Can you work these out from the model? Positions are in its coordinate system, mm. A direction names the side the tool comes from. Give positions to 0.01 mm unless a question says otherwise; leave off trailing zeros. Write each loop counter-clockwise with the first axis right and the second up, starting at its lowest first coordinate (ties: lowest second). Pieces come first, ordered by that corner, then holes. Notation, with made-up numbers: M 2,44 L 24,44 A14 cw 24,70 Z; hole C 51.5,73 d6. An arc over 180 degrees is marked long. Write each question's results on one line, items separated by ' | '.
from build123d import *

# Parameters (mm, degrees)
F1_R     = 2.5
F3_DEPTH = 35
F4_R     = 0.882114
F4_R_2   = 0.903169
F5_DEPTH = 25


with BuildPart() as f2:
    # F2: sweep along a path in F0
    with BuildLine(Plane.YZ) as f2_path:
        Line((0, 0), (0, 6.632662))
        ThreePointArc((0, 6.632662), (-1.942662, 11.322663), (-6.632662, 13.265325))
        Line((-6.632662, 13.265325), (-19.632662, 13.265325))
        ThreePointArc((-19.632662, 13.265325), (-24.322663, 15.207986), (-26.265325, 19.897987))
        Line((-26.265325, 19.897987), (-26.265325, 26.530649))
    # F1 (on Top) → F2 (sweep)
    with BuildSketch(Plane.XY):
        Circle(F1_R)
    sweep(path=f2_path.line)

    # F1 (on Top) → F3 (join)
    with BuildSketch(Plane.XY):
        Circle(F1_R)
    extrude(amount=-F3_DEPTH)

    # F4 (on face) → F5 (join)
    with BuildSketch(Plane(origin=(0, 0, -35), x_dir=(1, 0, 0), z_dir=(0, 0, -1))):
        with Locations((-1.37841, 0)):
            Circle(F4_R)
        with Locations((1.253585, 0)):
            Circle(F4_R_2)
    extrude(amount=F5_DEPTH)


solid = f2.part
Item 1: I want a section at A-A, the plane z = -36. Please give me the cut outline in (x, y).
Geometry says:
outline: C -1.38,0 d1.76; C 1.25,0 d1.81
Item 2: For faces 1 (the face through (0, 0, -35)), 2 (the face through (0, -26, 26.531)), which set-ups out of +Z, -Z, +X, -X, +Y, -Y let a thin tool reach every point of the face, with its end or its side?
Geometry says:
face 1: -Z | face 2: +Z, +X, -X, +Y, -Y
Item 3: I'm going to push flat-ended pins straight in: pin 1 (1 mm diameter, centred on x = 1, y = -11, fed in from -Z); pin 2 (1 mm diameter, centred on x = 2, z = -33.5, fed in from +Y); pin 3 (3 mm diameter, centred on y = -4.5, z = 2, fed in from -X). Where does each tip first touch, or does it pass through?
Geometry says:
pin 1: stops at z = 10.82 | pin 2: stops at y = 2 | pin 3: passes through
Item 4: Thinking about a two-plate mould opening in X: for faces 3 (the face through (-0.537, -0.265, -47.325)), 4 (the face through (1.058, 0.882, -47.325)), 5 (the face through (-1, 0, -60)), 6 (the face through (-0.54, -2.44, -13.89)), which applies, +X half, -X half, draft (parallel to the pull), parting line (faces both ways), or undercut?
Geometry says:
face 3: undercut | face 4: undercut | face 5: draft | face 6: parting line
Item 5: If I drill on line 1 (Z direction, x = 0.3, y = -12.5); line 2 (Y direction, x = 0.2, z = -25); line 3 (Y direction, x = 0, z = 21.5), over which ranges is the centre line in solid material (lowest first)? Write a range as from..to.
Geometry says:
line 1: z = 10.78..15.75 | line 2: y = -2.49..2.49 | line 3: y = -28.77..-23.77
